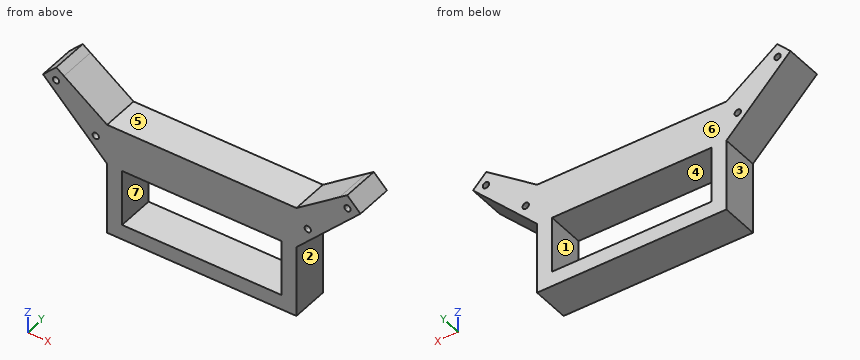
from build123d import *

# Parameters (mm, degrees)
BOSS_EXTRUDE1_DEPTH = 25.4


with BuildPart() as part:
    # Sketch3 → Boss-Extrude1 (new body)
    with BuildSketch(Plane(origin=(0, 0, 0), x_dir=(1, 0, 0), z_dir=(0, 1, 0))):
        Polygon((-53.975, -20.955), (-64.135, -31.115), (-64.135, -50.165), (64.135, -50.165), (64.135, -31.115), (53.975, -20.955), (53.975, -22.225), (-53.975, -22.225), align=None)
        Polygon((-64.135, 26.035), (-64.135, -22.565796173), (-64.135, -31.115), (-53.975, -20.955), (-53.975, 15.875), (-17.145, 15.875), (-6.985, 26.035), align=None)
        Polygon((6.985, 26.035), (-6.985, 26.035), (-17.145, 15.875), (17.145, 15.875), align=None)
        Polygon((64.135, 26.035), (6.985, 26.035), (17.145, 15.875), (53.975, 15.875), (53.975, -20.955), (64.135, -31.115), (64.135, -22.565796173), align=None)
        with BuildLine():
            Line((64.135, -22.565796173), (64.135, -31.115))
            Line((64.135, -31.115), (70.315405428, -37.295405428))
            ThreePointArc((70.315405428, -37.295405428), (72.668262499, -36.827393058), (74.001048969, -38.822048969))
            ThreePointArc((74.001048969, -38.822048969), (73.836704879, -39.648262499), (73.368692509, -40.348692509))
            Line((73.368692509, -40.348692509), (97.256173791, -64.236173791))
            ThreePointArc((97.256173791, -64.236173791), (99.609030862, -63.768161421), (100.941817332, -65.762817332))
            ThreePointArc((100.941817332, -65.762817332), (99.609030862, -67.757473242), (97.256173791, -67.289460872))
            Line((97.256173791, -67.289460872), (93.346419205, -71.199215458))
            Line((93.346419205, -71.199215458), (98.567291185, -74.9585996))
            Line((98.567291185, -74.9585996), (107.547547306, -65.978343479))
            Line((107.547547306, -65.978343479), (64.135, -22.565796173))
        make_face()
        with BuildLine():
            Line((64.135, -31.115), (64.135, -50.165))
            Line((64.135, -50.165), (93.346419205, -71.199215458))
            Line((93.346419205, -71.199215458), (97.256173791, -67.289460872))
            ThreePointArc((97.256173791, -67.289460872), (96.623817332, -65.762817332), (97.256173791, -64.236173791))
            Line((97.256173791, -64.236173791), (73.368692509, -40.348692509))
            ThreePointArc((73.368692509, -40.348692509), (70.315405428, -40.348692509), (70.315405428, -37.295405428))
            Line((70.315405428, -37.295405428), (64.135, -31.115))
        make_face()
        with BuildLine():
            Line((-64.135, -50.165), (-64.135, -31.115))
            Line((-64.135, -31.115), (-70.315405428, -37.295405428))
            ThreePointArc((-70.315405428, -37.295405428), (-69.847393058, -37.995835438), (-69.683048969, -38.822048969))
            ThreePointArc((-69.683048969, -38.822048969), (-71.015835438, -40.816704879), (-73.368692509, -40.348692509))
            Line((-73.368692509, -40.348692509), (-97.256173791, -64.236173791))
            ThreePointArc((-97.256173791, -64.236173791), (-96.788161421, -64.936603801), (-96.623817332, -65.762817332))
            ThreePointArc((-96.623817332, -65.762817332), (-96.788161421, -66.589030862), (-97.256173791, -67.289460872))
            Line((-97.256173791, -67.289460872), (-93.346419205, -71.199215458))
            Line((-93.346419205, -71.199215458), (-64.135, -50.165))
        make_face()
        with BuildLine():
            Line((-64.135, -31.115), (-64.135, -22.565796173))
            Line((-64.135, -22.565796173), (-107.547547306, -65.978343479))
            Line((-107.547547306, -65.978343479), (-98.567291185, -74.9585996))
            Line((-98.567291185, -74.9585996), (-93.346419205, -71.199215458))
            Line((-93.346419205, -71.199215458), (-97.256173791, -67.289460872))
            ThreePointArc((-97.256173791, -67.289460872), (-100.941817332, -65.762817332), (-97.256173791, -64.236173791))
            Line((-97.256173791, -64.236173791), (-73.368692509, -40.348692509))
            ThreePointArc((-73.368692509, -40.348692509), (-73.368692509, -37.295405428), (-70.315405428, -37.295405428))
            Line((-70.315405428, -37.295405428), (-64.135, -31.115))
        make_face()
    extrude(amount=BOSS_EXTRUDE1_DEPTH)


solid = part.part
Can you work these out from the model? Positions are in its coordinate system, mm. Face numbers are marked on the shaded views. A direction names the side the tool comes from. Round coordinates to 2 decimals unless told otherwise and drop trailing zeros. Write each loop counter-clockwise with the first axis right and the second up, starting at its lowest first coordinate (ties: lowest second). Pieces come first, ordered by that corner, then holes. Notation, with made-up numbers: (-23, -30) - (-18, -30) arc R28 cw to (-18, -2) - close; hole circle Ø7 at (-4.75, -38.75). An arc over 180 degrees is marked (long way). Write each question's results on one line, items separated by ' | '. Start each with the question number.
1) Which directions (+Z, -Z, +X, -X, +Y, -Y) give clear straight access to the entire face, cutting with the end or side of a thin tool? Please do the marked faces 5, 6 and 7.
2) Suppose I cut it at D-D (x = 83). List the corners of the cut face in (y, z) for me.
3) Suppose I cut it at C-C (z = -6). List the corners of the cut face in (x, y) for me (3 decimals), and give its area (3 significant figures).
4) For pin 1 Ø4 at (y, z) = (12, 34.5) entering from -X; pin 2 Ø10 at (y, z) = (11, 12) entering from -X (3 decimals); pin 3 Ø12.5 at (y, z) = (16.5, -5.5) entering from +X (3 decimals), each with a flat end and sliding along its axis, tell me the tip position at first contact or that it passes through.
5) Please list where these lines run through material, in increasing order: line 1 (Z direction, x = 6, y = 2) (3 decimals); line 2 (X direction, y = 6, z = 17.5) (3 decimals); line 3 (X direction, y = 3.5, z = 38).
6) We'd pull the mould along X, two halves only. Please class the marked faces 1, 2, 3 and 4: released by +X, released by -X, zero draft, split by the parting line, or undercut.
7) Suppose I cut it at A-A (x = 22). List the corners of the cut face in (y, z) for me (3 decimals), and give its area (3 significant figures).
8) Suppose I cut it at B-B (y = 12.25). List the corners of the cut face in (x, z) for me (3 decimals), and give its area (3 significant figures).
Here are the results:
1) face 5: +Z, +Y, -Y | face 6: +Z, -Z, +X, -X, +Y | face 7: +Y, -Y
2) outline: (0, 41.43) - (25.4, 41.43) - (25.4, 63.75) - (0, 63.75) - close
3) outline: (-64.135, 0) - (-53.975, 0) - (-53.975, 25.4) - (-64.135, 25.4) - close; (53.975, 0) - (64.135, 0) - (64.135, 25.4) - (53.975, 25.4) - close | area: 516 mm2
4) pin 1: stops at x = -78.07 | pin 2: stops at x = -64.135 | pin 3: stops at x = 64.135
5) line 1: z = -26.035 to -15.875, 22.225 to 50.165 | line 2: x = -64.135 to -53.975, 53.975 to 64.135 | line 3: x = -79.57 to -73.84, -69.85 to 69.85, 73.84 to 79.57
6) face 1: undercut | face 2: released by +X | face 3: released by -X | face 4: undercut
7) outline: (0, -26.035) - (25.4, -26.035) - (25.4, -15.875) - (0, -15.875) - close; (0, 22.225) - (25.4, 22.225) - (25.4, 50.165) - (0, 50.165) - close | area: 968 mm2
8) outline: (-107.548, 65.978) - (-64.135, 22.566) - (-64.135, -26.035) - (64.135, -26.035) - (64.135, 22.566) - (107.548, 65.978) - (98.567, 74.959) - (64.135, 50.165) - (-64.135, 50.165) - (-98.567, 74.959) - close; hole circle Ø4.318 at (-98.783, 65.763); hole circle Ø4.318 at (-71.842, 38.822); hole (-53.975, -15.875) - (53.975, -15.875) - (53.975, 22.225) - (-53.975, 22.225) - close; hole circle Ø4.318 at (71.842, 38.822); hole circle Ø4.318 at (98.783, 65.763) | area: 7,330 mm2
